For this review, use the dimensioned drawing (mm, ordinates from the lowest corner) and the shaded views. A direction names the side the tool comes from. Give positions to 0.01 mm unless a question says otherwise; leave off trailing zeros. Write each loop counter-clockwise with the first axis right and the second up, starting at its lowest first coordinate (ties: lowest second). Pieces come first, ordered by that corner, then holes.
1) Wall thickness on line 1 along Z through (x, y) = (20, 24.5); line 2 along Y through (x, z) = (1.5, 6.5); line 3 along Z through (x, y) = (4.5, 22.25): over which ranges is each line inside the solid? List them lowest first.
2) Draft analysis for pull direction Y (two halves, no side actions). For the marked faces 1, 2 and 3, state which applies: pulls with the +Y half, pulls with the -Y half, needs draft (parallel to the pull), parting line crosses it, or undercut.
3) We need section B-B on x = 4.5. Give the boundary of the cut face in (y, z), and give its area (3 significant figures).
4) We need section D-D on x = 11.5. Give the boundary of the cut face in (y, z).
5) We need section C-C on z = 8.5. Give the boundary of the cut face in (x, y), and give its area (3 significant figures).
6) We need section A-A on y = 24.5. Give the boundary of the cut face in (x, z).
7) For P1, Ø1.8, axis at y = 24.5, z = 14.5, coming from the +X side; P2, Ø6.5, axis at x = 4.5, z = 8.5, coming from the +Y side; P3, Ø1, axis at y = 10.5, z = 10.5, coming from the -X side; P4, Ø7, axis at x = 4.5, z = 8.5, coming from the -Y side, all flat-tipped, find the tip position at first contact; note any pin that passes through.
8) Machinability: for the marked faces 4, 5, 6 and 7, which of the approach directions +Z, -Z, +X, -X, +Y, -Y give a long, thin tool a straight path to every point of the face, cutting with its end or side? Answer none if there is none.
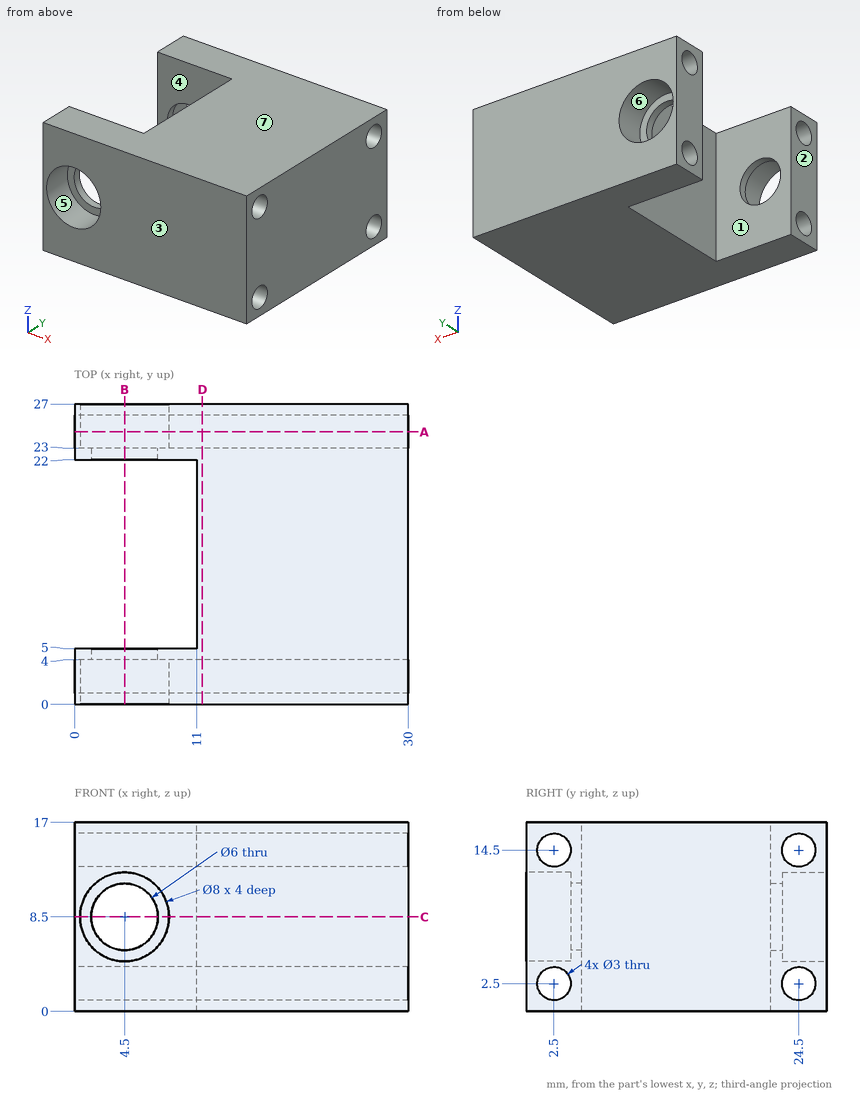
Results list:
1. line 1: z = 0 to 1, 4 to 13, 16 to 17
1. line 2: y = 4 to 5, 22 to 23
1. line 3: z = 0 to 5.5, 11.5 to 17
2. face 1: undercut
2. face 2: needs draft
2. face 3: pulls with the -Y half
3. outline: (0, 0) - (5, 0) - (5, 5.5) - (4, 5.5) - (4, 4.5) - (0, 4.5) - close; (0, 12.5) - (4, 12.5) - (4, 11.5) - (5, 11.5) - (5, 17) - (0, 17) - close; (22, 0) - (27, 0) - (27, 4.5) - (23, 4.5) - (23, 5.5) - (22, 5.5) - close; (22, 11.5) - (23, 11.5) - (23, 12.5) - (27, 12.5) - (27, 17) - (22, 17) - close; hole circle Ø3 at (2.5, 2.5); hole circle Ø3 at (2.5, 14.5); hole circle Ø3 at (24.5, 2.5); hole circle Ø3 at (24.5, 14.5)
3. area: 65.7 mm2
4. outline: (0, 0) - (27, 0) - (27, 17) - (0, 17) - close; hole circle Ø3 at (2.5, 2.5); hole circle Ø3 at (2.5, 14.5); hole circle Ø3 at (24.5, 2.5); hole circle Ø3 at (24.5, 14.5)
5. outline: (0, 0) - (0.5, 0) - (0.5, 4) - (1.5, 4) - (1.5, 5) - (0, 5) - close; (0, 22) - (1.5, 22) - (1.5, 23) - (0.5, 23) - (0.5, 27) - (0, 27) - close; (7.5, 4) - (8.5, 4) - (8.5, 0) - (30, 0) - (30, 27) - (8.5, 27) - (8.5, 23) - (7.5, 23) - (7.5, 22) - (11, 22) - (11, 5) - (7.5, 5) - close
5. area: 547 mm2
6. outline: (0, 0) - (30, 0) - (30, 1) - (0, 1) - close; (0, 4) - (30, 4) - (30, 13) - (0, 13) - close; (0, 16) - (30, 16) - (30, 17) - (0, 17) - close; hole circle Ø8 at (4.5, 8.5)
7. P1: passes through
7. P2: stops at y = 23
7. P3: stops at x = 11
7. P4: stops at y = 4
8. face 4: +Z, -Z, -X
8. face 5: -Y
8. face 6: +Y
8. face 7: +Z, +X, -X, +Y, -Y
